```python
from build123d import *

# Parameters (mm, degrees)
EXTRUDE_1_DEPTH     = 5
CHAMFER_1_SIZE      = 0.5
FILLET_1_R          = 1
SKETCH_3_R          = 0.8
CUT_EXTRUDE_1_DEPTH = 4


with BuildPart() as part:
    # 草图2 → 凸台-拉伸1 (new body)
    with BuildSketch(Plane.XY):
        Polygon((-3.6, 0), (-3.6, -6.8), (3.6, -6.8), (3.6, 0), (6.6, 0), (6.6, -9.8), (-6.6, -9.8), (-6.6, 0), align=None)
    extrude(amount=EXTRUDE_1_DEPTH)

    # 倒角1
    chamfer_1_edges = [part.edges().sort_by_distance(p)[0] for p in [
        (-3.6, 0, 2.5),
        (3.6, 0, 2.5),
    ]]
    chamfer(chamfer_1_edges, length=CHAMFER_1_SIZE)

    # 圆角1
    fillet_1_edges = [part.edges().sort_by_distance(p)[0] for p in [
        (6.6, 0, 2.5),
        (6.6, -9.8, 2.5),
        (-6.6, -9.8, 2.5),
        (-6.6, 0, 2.5),
    ]]
    fillet(fillet_1_edges, radius=FILLET_1_R)

    # 草图3 → 切除-拉伸1 (cut)
    with BuildSketch(Plane(origin=(0, -6.8, 0), x_dir=(1, 0, 0), z_dir=(0, 1, 0))):
        with Locations(Location((0, -2.5, 0), (0, 0, 180))):
            Circle(SKETCH_3_R)
    extrude(amount=-CUT_EXTRUDE_1_DEPTH, mode=Mode.SUBTRACT)


solid = part.part
```
For this review, take the finished solid that the model builds, in its own axes (mm). A direction names the side the tool comes from. Round coordinates to 2 decimals unless told otherwise and drop trailing zeros. Write each loop counter-clockwise with the first axis right and the second up, starting at its lowest first coordinate (ties: lowest second). Pieces come first, ordered by that corner, then holes. Notation, with made-up numbers: (49.25, -3) - (105.25, -3) arc R21 ccw to (105.25, 5) - close; hole circle Ø8 at (21, -37). An arc over 180 degrees is marked (long way). Answer as a JSON object with one key per item and string values.
1. We need section D-D on z = 4.5. Give the boundary of the cut face in (x, y).
Response values:
{"outline": "(-6.6, -8.8) arc R1 ccw to (-5.6, -9.8) - (5.6, -9.8) arc R1 ccw to (6.6, -8.8) - (6.6, -1) arc R1 ccw to (5.6, 0) - (4.1, 0) - (3.6, -0.5) - (3.6, -6.8) - (-3.6, -6.8) - (-3.6, -0.5) - (-4.1, 0) - (-5.6, 0) arc R1 ccw to (-6.6, -1) - close"}
2. To check wall thickness, follow line 1 along X through (y, z) = (-6.75, 4.6); line 2 along Z through (x, y) = (0, -7.7); line 3 along Y through (x, z) = (-1.5, 3.95). State the ranges of each line that lie inside material, in increasing order.
Response values:
{"line 1": "x = -6.6 to -3.6, 3.6 to 6.6", "line 2": "z = 0 to 1.7, 3.3 to 5", "line 3": "y = -9.8 to -6.8"}
3. Draft analysis for pull direction X (two halves, no side actions). For faces 1 (the face through (5, 0, 2)), 2 (the face through (-6.315, -9.499, 2.535)), 3 (the face through (-3.6, -4, 2)), state which applies: +X half, -X half, draft (parallel to the pull), parting line (faces both ways), or undercut.
Response values:
{"face 1": "draft", "face 2": "-X half", "face 3": "undercut"}
4. We need section A-A on y = -6.5. Give the boundary of the cut face in (x, z), then the cut area to 3 significant figures.
Response values:
{"outline": "(-6.6, 0) - (-3.6, 0) - (-3.6, 5) - (-6.6, 5) - close; (3.6, 0) - (6.6, 0) - (6.6, 5) - (3.6, 5) - close", "area": "30.0 mm2"}
5. We need section C-C on z = 2.5. Give the boundary of the cut face in (x, y).
Response values:
{"outline": "(-6.6, -8.8) arc R1 ccw to (-5.6, -9.8) - (-0.8, -9.8) - (-0.8, -6.8) - (-3.6, -6.8) - (-3.6, -0.5) - (-4.1, 0) - (-5.6, 0) arc R1 ccw to (-6.6, -1) - close; (0.8, -9.8) - (5.6, -9.8) arc R1 ccw to (6.6, -8.8) - (6.6, -1) arc R1 ccw to (5.6, 0) - (4.1, 0) - (3.6, -0.5) - (3.6, -6.8) - (0.8, -6.8) - close"}
6. Tool access review of faces 4 (the face through (3.6, -4, 2)), 5 (the face through (0.17, -8.28, 1.72)): name each direction out of +Z, -Z, +X, -X, +Y, -Y from which nothing blocks a thin tool from reaching the whole face with its end or side.
Response values:
{"face 4": "+Z, -Z, +Y", "face 5": "+Y, -Y"}
7. We need section B-B on x = 0. Give the boundary of the cut face in (y, z).
Response values:
{"outline": "(-9.8, 0) - (-6.8, 0) - (-6.8, 1.7) - (-9.8, 1.7) - close; (-9.8, 3.3) - (-6.8, 3.3) - (-6.8, 5) - (-9.8, 5) - close"}
